```python
from build123d import *

# Parameters (mm, degrees)
BOSS_EXTRUDE1_DEPTH     = 2
EXTRUDE_THIN2_START     = 50
EXTRUDE_THIN2_DEPTH     = 50
RIB2_START              = -2
RIB2_OUTLINE_W          = 51
RIB2_OUTLINE_H          = 3
RIB2_DEPTH              = 4
RIB14_START             = -2
RIB14_OUTLINE_W         = 50
RIB14_OUTLINE_H         = 1
RIB14_DEPTH             = 4
LPATTERN1_COUNT         = 3
LPATTERN1_PITCH         = 53
MIRROR1_START           = -2
MIRROR1_COPY_1_SKETCH_W = 50
MIRROR1_COPY_1_SKETCH_H = 1
MIRROR1_COPY_1_DEPTH    = 4
MIRROR1_COPY_2_SKETCH_W = 50
MIRROR1_COPY_2_SKETCH_H = 1
MIRROR1_COPY_2_DEPTH    = 4
SKETCH6_R               = 1
CUT_EXTRUDE1_DEPTH      = 10


# Read off the part's stored shape, not the designer's step: Rib2, Rib14
with BuildPart() as part:
    # Sketch2 → Boss-Extrude1 (new body)
    with BuildSketch(Plane(origin=(0, 0, 0), x_dir=(0, 0, -1), z_dir=(1, 0, 0))):
        with BuildLine():
            Line((30, -70), (-30, -70))
            Line((-30, -70), (-30, 40))
            ThreePointArc((-30, 40), (0, 70), (30, 40))
            Line((30, 40), (30, -70))
        make_face()
    extrude(amount=BOSS_EXTRUDE1_DEPTH)

    # Sketch5 → Extrude-Thin2 (add)
    with BuildSketch(Plane.ZY.offset(EXTRUDE_THIN2_START)):
        with BuildLine():
            Line((-30, 40), (-30, -70))
            Line((-30, -70), (30, -70))
            Line((30, -70), (30, 40))
            ThreePointArc((30, 40), (0, 70), (-30, 40))
        make_face()
        with BuildLine():
            Line((-28, 40), (-28, -68))
            Line((-28, -68), (28, -68))
            Line((28, -68), (28, 40))
            ThreePointArc((28, 40), (0, 68), (-28, 40))
        make_face(mode=Mode.SUBTRACT)
    extrude(amount=-EXTRUDE_THIN2_DEPTH)

    # Rib2 outline → Rib2 (add)
    with BuildSketch(Plane.XY.offset(RIB2_START)):
        with Locations((-24.5, 67.5)):
            Rectangle(RIB2_OUTLINE_W, RIB2_OUTLINE_H)
    extrude(amount=RIB2_DEPTH)

    # Rib14 outline → Rib14 (add)
    with BuildSketch(Plane(origin=(0, 40, 0), x_dir=(1, 0, 0), z_dir=(0, 1, 0)).offset(RIB14_START)):
        with Locations((-25, 27.5)):
            Rectangle(RIB14_OUTLINE_W, RIB14_OUTLINE_H)
    rib14 = extrude(amount=RIB14_DEPTH)

    # LPattern1: Rib14 ×3
    with Locations(*[(0, -i * LPATTERN1_PITCH, 0) for i in range(1, LPATTERN1_COUNT)]):
        add(rib14)

    # Mirror1: Rib14 across plane
    add(rib14.mirror(Plane.XY))

    # Mirror1 copy 1 sketch → Mirror1 copy 1 (add)
    with BuildSketch(Plane(origin=(0, -13, 0), x_dir=(1, 0, 0), z_dir=(0, 1, 0)).offset(MIRROR1_START)):
        with Locations((-25, -27.5)):
            Rectangle(MIRROR1_COPY_1_SKETCH_W, MIRROR1_COPY_1_SKETCH_H)
    extrude(amount=MIRROR1_COPY_1_DEPTH)

    # Mirror1 copy 2 sketch → Mirror1 copy 2 (add)
    with BuildSketch(Plane(origin=(0, -66, 0), x_dir=(1, 0, 0), z_dir=(0, 1, 0)).offset(MIRROR1_START)):
        with Locations((-25, -27.5)):
            Rectangle(MIRROR1_COPY_2_SKETCH_W, MIRROR1_COPY_2_SKETCH_H)
    extrude(amount=MIRROR1_COPY_2_DEPTH)

    # Sketch6 → Cut-Extrude1 (cut)
    with BuildSketch(Plane.ZY.offset(50)):
        with Locations((0, 68.5)):
            Circle(SKETCH6_R)
        with Locations((-28.5, 40)):
            Circle(SKETCH6_R)
        with Locations((28.5, 40)):
            Circle(SKETCH6_R)
        with Locations((28.5, -13)):
            Circle(SKETCH6_R)
        with Locations((28.5, -66)):
            Circle(SKETCH6_R)
        with Locations((-28.5, -13)):
            Circle(SKETCH6_R)
        with Locations((-28.5, -66)):
            Circle(SKETCH6_R)
    extrude(amount=-CUT_EXTRUDE1_DEPTH, mode=Mode.SUBTRACT)


solid = part.part
```
The model under review builds one solid part; all positions refer to its coordinate system, in mm. A direction names the side the tool comes from. Give positions to 0.01 mm unless a question says otherwise; leave off trailing zeros. Write each loop counter-clockwise with the first axis right and the second up, starting at its lowest first coordinate (ties: lowest second). Pieces come first, ordered by that corner, then holes. Notation, with made-up numbers: (48.25, 81) - (81.25, 81) arc R24 cw to (81.25, 95) - close; hole circle Ø2 at (29, 63). An arc over 180 degrees is marked (long way). Answer in a Markdown table with one row per item. Add a question column.
1. Wall thickness on line 1 along Z through (x, y) = (-43, -66); line 2 along Z through (x, y) = (-12, -47); line 3 along X through (y, z) = (53.5, 10.5): over which ranges is each line inside the solid? List them lowest first. Write a range as [from, to].
2. We need section D-D on x = -47. State how many separate pieces and enclosed holes the cut face has, then the cut area to 3 significant figures.
3. We need section A-A on y = 29.5. Write out the cut boundary in (x, z).
4. Draft analysis for pull direction Y (two halves, no side actions). For faces 3 (the flat face through (-25, 13, 28)), 4 (the cylindrical face through (-24.364, 69.993, 0.66)), 5 (the flat face through (-50, 5, 29)), state which applies: +Y half, -Y half, draft (parallel to the pull), parting line (faces both ways), or undercut.
5. We need section C-C on z = -15.5. Write out the cut boundary in (x, y).
6. Insertion check: P1, Ø1.8, axis at y = 68.5, z = 0, coming from the -X side; P2, Ø2, axis at y = -12, z = 11.5, coming from the -X side; P3, Ø1, axis at x = -29.5, z = -20.5, coming from the +Y side; P4, Ø4.5, axis at x = -27.5, y = 41, coming from the -Z side. Each pin has a flat end and moves straight along its axis. Give the tip position at first contact, or say it passes through.
7. Tool access review of faces 1 (the flat face through (-25, 14, -28)), 2 (the flat face through (2, 1, 0)): name each direction out of +Z, -Z, +X, -X, +Y, -Y from which nothing blocks a thin tool from reaching the whole face with its end or side.
Ans:
| question | item | result |
|---|---|---|
| 1 | line 1 | z = [-30, -29.5], [-27.5, -27], [27, 27.5], [29.5, 30] |
| 1 | line 2 | z = [-30, -28], [28, 30] |
| 1 | line 3 | x = [0, 2] |
| 2 | separate pieces | 1 |
| 2 | enclosed holes | 8 |
| 2 | area | 744 mm^2 |
| 3 | outline | (-50, -30) - (2, -30) - (2, 30) - (-50, 30) - (-50, 28) - (0, 28) - (0, -28) - (-50, -28) - close |
| 4 | face 3 | undercut |
| 4 | face 4 | +Y half |
| 4 | face 5 | draft |
| 5 | outline | (-50, -70) - (2, -70) - (2, 65.69) - (-50, 65.69) - (-50, 63.32) - (0, 63.32) - (0, -68) - (-50, -68) - close |
| 6 | P1 | stops at x = -40 |
| 6 | P2 | stops at x = 0 |
| 6 | P3 | stops at y = 62.36 |
| 6 | P4 | stops at z = -30 |
| 7 | face 1 | -X |
| 7 | face 2 | +Z, -Z, +X, +Y, -Y |
